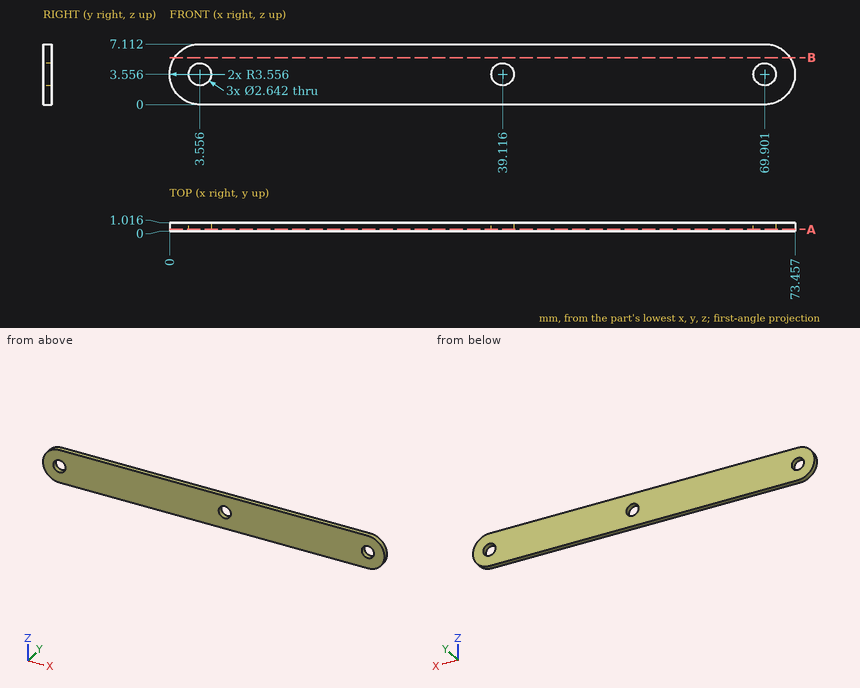
Source: three-view drawing plus pictorial views. Frame: mm from the lowest corner of the part. Round coordinates to 2 decimals unless told otherwise and drop trailing zeros. Loops run counter-clockwise (first coordinate to the right, second up) from the corner with the lowest first, then second, coordinate; pieces in that order, holes last. Notation, with made-up numbers: M 11,19 L 55,19 A8 cw 55,31 Z; hole C 1,-21.5 d10. An arc over 180 degrees is marked long. Put each result on its own line as item: value.
(1) Ray query, line 1 (X direction, y = 0.35, z = 2.75) (1 decimal); line 2 (X direction, y = 0.3, z = 4) (1 decimal); line 3 (X direction, y = 0.55, z = 6.5) (1 decimal). Return the intervals inside material, ascending. Write a range as [from, to].
Solutions:
line 1: [0.1, 2.5], [4.6, 38.1], [40.2, 68.9], [70.9, 73.4]
line 2: [0, 2.3], [4.8, 37.9], [40.4, 68.7], [71.1, 73.4]
line 3: [1.6, 71.9]
(2) First-contact query: pin 1 (1 mm diameter, centred on x = 18.5, z = 4.5, fed in from -Y). Flat tip, straight axial feed; report the tip coordinate or a pass-through.
Solutions:
pin 1: y = 0
(3) Section A-A, the plane y = 0.2. Return loops of the section in (x, z) (1 decimal).
Solutions:
outline: M 3.6,0 L 69.9,0 A3.6 ccw 69.9,7.1 L 3.6,7.1 A3.6 ccw Z; hole C 3.6,3.6 d2.6; hole C 39.1,3.6 d2.6; hole C 69.9,3.6 d2.6
(4) Section B-B, the plane z = 5.5. Return loops of the section in (x, y).
Solutions:
outline: M 0.58,0 L 72.88,0 L 72.88,1.02 L 0.58,1.02 Z
